The model under review builds one solid part; all positions refer to its coordinate system, in mm. A direction names the side the tool comes from. Give positions to 0.01 mm unless a question says otherwise; leave off trailing zeros. Order: outer loops, then holes, each group sorted by start corner. A loop starts at its lowest first (then second) coordinate and runs counter-clockwise, first axis right, second up.
```python
from build123d import *

# Parameters (mm, degrees)
F0_R     = 19.694794
F1_DEPTH = 55.372
F4_DEPTH = 114.046
F6_DEPTH = 254


with BuildPart() as f1:
    # F0 (on Top) → F1 (new body)
    with BuildSketch(Plane.XY):
        Circle(F0_R)
    extrude(amount=F1_DEPTH)

    # F3 (on offset) → F4 (cut)
    with BuildSketch(Plane.XZ.offset(62.738)):
        Polygon((23.87774, 61.791748), (11.794434, 56.214053), (11.794434, 44.826049), (23.87774, 44.826049), align=None)
    extrude(amount=-F4_DEPTH, mode=Mode.SUBTRACT)

    # F5 (on offset) → F6 (cut)
    with BuildSketch(Plane.XZ.offset(62.738)):
        Polygon((-14.930949, 19.263754), (-14.930949, 14.383911), (-14.930949, 4.391609), (14.583289, 4.391609), (14.583289, 19.263754), align=None)
        Polygon((8.540357, 56.446675), (0, 56.446675), (-21.901777, 57.607204), (-21.901777, 20.426836), align=None)
    extrude(amount=-F6_DEPTH, mode=Mode.SUBTRACT)


solid = f1.part
```
Item 1: Take a section at A-A (y = 0). Give the boundary of the cut face in (x, z), and give its area (3 significant figures).
Values found:
outline: (-19.69, 0) - (19.69, 0) - (19.69, 44.83) - (11.79, 44.83) - (11.79, 55.37) - (7.63, 55.37) - (-19.69, 23.04) - close; hole (-14.93, 4.39) - (14.58, 4.39) - (14.58, 19.26) - (-14.93, 19.26) - close
area: 1,220 mm2
Item 2: Draft analysis for pull direction Z (two halves, no side actions). For faces 1 (the flat face through (0, 0, 4.392)), 2 (the flat face through (15, 0, 44.826)), 3 (the flat face through (11.794, 0, 50)), state which applies: released by +Z, released by -Z, zero draft, split by the parting line, or undercut.
Values found:
face 1: undercut
face 2: released by +Z
face 3: zero draft
Item 3: For faces 4 (the flat face through (-3.19, -0.28, 42.57)), 5 (the flat face through (14.583, 0, 12)), list the 3-axis set-ups (+Z, -Z, +X, -X, +Y, -Y) from which the entire face can be reached by the end or side of a thin tool; tool diameter is ignored.
Values found:
face 4: +Z, -X, +Y, -Y
face 5: +Y, -Y
Item 4: Take a section at B-B (x = 1.5). Give the boundary of the cut face in (y, z).
Values found:
outline: (-19.64, 0) - (19.64, 0) - (19.64, 4.39) - (-19.64, 4.39) - close; (-19.64, 19.26) - (19.64, 19.26) - (19.64, 48.12) - (-19.64, 48.12) - close
Item 5: Clearance check with flat-ended pins moving along their axes: pin 1 Ø1.5 at (y, z) = (11.5, 35.5) entering from +X; pin 2 Ø10 at (y, z) = (-11.5, 9) entering from -X; pin 3 Ø2 at (x, z) = (10.5, 26) entering from +Y. State where each tip first meets the part, or that it passes through.
Values found:
pin 1: stops at x = 16.5
pin 2: stops at x = -18.59
pin 3: stops at y = 17.25
Item 6: Take a section at C-C (z = 12). Give the boundary of the cut face in (x, y).
Values found:
outline: (-14.93, -12.84) - (-14.93, 12.84) arc R19.69 ccw to start; (14.58, -13.24) arc R19.69 ccw to (14.58, 13.24) - close
Item 7: Take a section at D-D (y = 14.5). Give the boundary of the cut face in (x, z).
Values found:
outline: (-13.33, 0) - (13.33, 0) - (13.33, 4.39) - (-13.33, 4.39) - close; (-13.33, 19.26) - (13.33, 19.26) - (13.33, 44.83) - (11.79, 44.83) - (11.79, 55.37) - (7.63, 55.37) - (-13.33, 30.57) - close
Item 8: For line 1 (Z direction, x = 14, y = -3.5); line 2 (Z direction, x = 16.5, y = 10.5); line 3 (Z direction, x = 4, y = 2.5), list the stretches that pass through material, from the lowest coordinate up.
Values found:
line 1: z = 0 to 4.39, 19.26 to 44.83
line 2: z = 0 to 44.83
line 3: z = 0 to 4.39, 19.26 to 51.07
